Build history of the part. All positions in model axes, mm. Face numbers are marked on the shaded views. A direction names the side the tool comes from. Round coordinates to 2 decimals unless told otherwise and drop trailing zeros. Order: outer loops, then holes, each group sorted by start corner. A loop starts at its lowest first (then second) coordinate and runs counter-clockwise, first axis right, second up. Notation, with made-up numbers: M 37.25,54.25 L 92.25,54.25 A6 cw 92.25,59.25 Z; hole C 31.25,43 d2. An arc over 180 degrees is marked long. One line per item, written item: value. Start each with the question number.
Item 1: Band-saw the part on C-C, the plane z = 5.5. Write the cut outline in (x, y).
Item 2: Probe L1, parallel to X at y = 46, z = 9.75; L2, parallel to Z at x = 77, y = 47; L3, parallel to X at y = 39, z = 13. List the from-to ranges inside material, lowest first.
Item 3: Band-saw the part on D-D, the plane y = 62. Write the cut outline in (x, z), then the cut area to 3 significant figures.
Item 4: Tool access for the marked faces 1 and 2: list every direction of +Z, -Z, +X, -X, +Y, -Y with a clear straight run to the whole face (end or side of a thin tool).
Item 5: Pin check, flat tips, straight feed: pin 1 (1 mm diameter, centred on y = 57.5, z = 9, fed in from +X); pin 2 (1 mm diameter, centred on x = 46.5, z = 3, fed in from -Y); pin 3 (1 mm diameter, centred on x = 65, z = 6.5, fed in from -Y). Stop position of each tip, or through.
Item 6: Band-saw the part on A-A, the plane x = 27. Write the cut outline in (y, z).
Item 7: Band-saw the part on B-B, the plane y = 33.5. Write the cut outline in (x, z).
Item 8: Two-plate mould, pull along Y, no slides. Class the marked faces 3, 4 and 5: +Y half, -Y half, draft (parallel to the pull), parting line (faces both ways), or undercut.
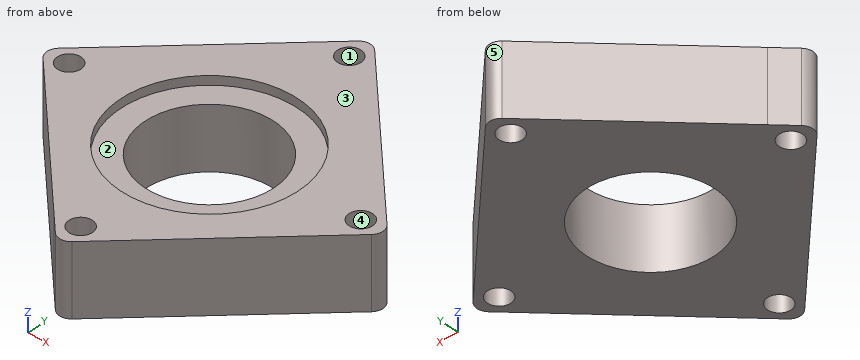
```python
from build123d import *

# Parameters (mm, degrees)
SKETCH1_R           = 14.5
SKETCH1_R_2         = 2.655602963
BOSS_EXTRUDE1_DEPTH = 16
SKETCH2_R           = 20
CUT_EXTRUDE1_DEPTH  = 2


with BuildPart() as part:
    # Sketch1 → Boss-Extrude1 (new body)
    with BuildSketch(Plane.XY):
        with BuildLine():
            Line((96.456721684, 48.36687177), (64.849048565, 79.974544889))
            Line((64.849048565, 79.974544889), (60.818539912, 84.005053542))
            ThreePointArc((60.818539912, 84.005053542), (58.909351603, 84.795865233), (57.000163293, 84.005053542))
            Line((57.000163293, 84.005053542), (25.392490174, 52.397380423))
            Line((25.392490174, 52.397380423), (21.361981522, 48.36687177))
            ThreePointArc((21.361981522, 48.36687177), (20.571169831, 46.457683461), (21.361981522, 44.548495152))
            Line((21.361981522, 44.548495152), (52.969654641, 12.940822033))
            Line((52.969654641, 12.940822033), (57.000163293, 8.91031338))
            ThreePointArc((57.000163293, 8.91031338), (58.909351603, 8.119501689), (60.818539912, 8.91031338))
            Line((60.818539912, 8.91031338), (92.426213031, 40.517986499))
            Line((92.426213031, 40.517986499), (96.456721684, 44.548495152))
            ThreePointArc((96.456721684, 44.548495152), (97.247533374, 46.457683461), (96.456721684, 48.36687177))
        make_face()
        with Locations((58.909351603, 45.077265813)):
            Circle(SKETCH1_R, mode=Mode.SUBTRACT)
        with Locations((58.909351603, 13.124669796)):
            Circle(SKETCH1_R_2, mode=Mode.SUBTRACT)
        with Locations((92.242365268, 46.457683461)):
            Circle(SKETCH1_R_2, mode=Mode.SUBTRACT)
        with Locations((58.909351603, 79.790697126)):
            Circle(SKETCH1_R_2, mode=Mode.SUBTRACT)
        with Locations((25.576337937, 46.457683461)):
            Circle(SKETCH1_R_2, mode=Mode.SUBTRACT)
    extrude(amount=BOSS_EXTRUDE1_DEPTH)

    # Sketch2 → Cut-Extrude1 (cut)
    with BuildSketch(Plane.XY.offset(16)):
        with Locations((58.909351603, 45.077265813)):
            Circle(SKETCH2_R)
    extrude(amount=-CUT_EXTRUDE1_DEPTH, mode=Mode.SUBTRACT)


solid = part.part
```
Output:
1. outline: M 21.36,44.55 L 57,8.91 A2.7 ccw 60.82,8.91 L 96.46,44.55 A2.7 ccw 96.46,48.37 L 60.82,84.01 A2.7 ccw 57,84.01 L 21.36,48.37 A2.7 ccw Z; hole C 25.58,46.46 d5.31; hole C 58.91,45.08 d29; hole C 58.91,13.12 d5.31; hole C 58.91,79.79 d5.31; hole C 92.24,46.46 d5.31
2. L1: x = 20.61 to 22.96, 28.19 to 44.44, 73.38 to 89.63, 94.86 to 97.21
2. L2: z = 0 to 14
2. L3: x = 26.91 to 45.74, 72.07 to 90.91
3. outline: M 35,0 L 82.82,0 L 82.82,16 L 69.57,16 L 69.57,14 L 48.25,14 L 48.25,16 L 35,16 Z
3. area: 723 mm²
4. face 1: +Z, -Z
4. face 2: +Z
5. pin 1: stops at x = 87.82
5. pin 2: stops at y = 18.91
5. pin 3: stops at y = 12.59
6. outline: M 38.91,0 L 44.22,0 L 44.22,16 L 38.91,16 Z; M 48.7,0 L 54,0 L 54,16 L 48.7,16 Z
7. outline: M 32.41,0 L 50.18,0 L 50.18,14 L 42.6,14 L 42.6,16 L 32.41,16 Z; M 67.64,0 L 85.41,0 L 85.41,16 L 75.22,16 L 75.22,14 L 67.64,14 Z
8. face 3: draft
8. face 4: undercut
8. face 5: +Y half
